from build123d import *

# Parameters (mm, degrees)
SKETCH1_R           = 50
SKETCH1_R_2         = 40
BOSS_EXTRUDE1_DEPTH = 10
SKETCH2_R           = 2
BOSS_EXTRUDE2_DEPTH = 33
CIRPATTERN1_COUNT   = 4


with BuildPart() as part:
    # Sketch1 → Boss-Extrude1 (new body)
    with BuildSketch(Plane(origin=(0, 0, 0), x_dir=(1, 0, 0), z_dir=(0, 1, 0))):
        with Locations(Location((0, 0, 0), (0, 0, 270))):
            Circle(SKETCH1_R)
        with Locations(Location((0, 0, 0), (0, 0, 270))):
            Circle(SKETCH1_R_2, mode=Mode.SUBTRACT)
    extrude(amount=BOSS_EXTRUDE1_DEPTH)

    # Sketch2 → Boss-Extrude2 (add)
    with BuildSketch(Plane(origin=(0, 10, 0), x_dir=(1, 0, 0), z_dir=(0, 1, 0))):
        with Locations(Location((0, 45, 0), (0, 0, 270))):
            Circle(SKETCH2_R)
    boss_extrude2 = extrude(amount=BOSS_EXTRUDE2_DEPTH)

    # CirPattern1: Boss-Extrude2 ×4 about axis
    cirpattern1_axis = Axis((0, 0, 0), (0, 1, 0))
    for i in range(1, CIRPATTERN1_COUNT):
        add(boss_extrude2.rotate(cirpattern1_axis, i * 360 / CIRPATTERN1_COUNT))


solid = part.part
Geometry: final body of the model. Coordinates: model frame, mm. A direction names the side the tool comes from. Round coordinates to 2 decimals unless told otherwise and drop trailing zeros. Loops run counter-clockwise (first coordinate to the right, second up) from the corner with the lowest first, then second, coordinate; pieces in that order, holes last. Notation, with made-up numbers: M -36,41.5 L 8,41.5 A34 ccw 8,77.5 Z; hole C -6.5,-40 d6. An arc over 180 degrees is marked long. Put each result on its own line as item: value. Start each with the question number.
(1) Draft query along X for faces 1 (the face through (0, 43, -45)), 2 (the face through (0, 26, 47)), 3 (the face through (-47, 26, 0)). Return one class per face: +X half, -X half, draft (parallel to the pull), parting line (faces both ways), or undercut.
(2) Section query B-B (z = 0). Return loops of the section in (x, y).
(3) Material intervals for line 1 along X through (y, z) = (5, 0); line 2 along Y through (x, z) = (-21, -36); line 3 along Z through (x, y) = (-25.5, 6), sorted ascending. Write a range as [from, to].
(4) Set-up query: faces 4 (the face through (0, 26, -47)), 5 (the face through (-45, 43, 0)). Return all of +Z, -Z, +X, -X, +Y, -Y with unobstructed straight access to the full face (end or side cutting, diameter ignored); none if empty.
(5) Contact query for flat-ended pins moving along their axis: pin 1 Ø5 at (y, z) = (12, -22.5) entering from -X; pin 2 Ø12 at (x, z) = (2.5, -30) entering from -Y; pin 3 Ø4 at (y, z) = (6, 19.5) entering from +X. Output: stop coordinate, or through.
(6) Section query D-D (z = 27.5). Return loops of the section in (x, y).
(7) Section query C-C (y = 14.5). Return loops of the section in (x, z).
(8) Section query A-A (x = 0). Return loops of the section in (y, z).
Findings below:
1. face 1: draft
1. face 2: parting line
1. face 3: undercut
2. outline: M -50,0 L -40,0 L -40,10 L -43,10 L -43,43 L -47,43 L -47,10 L -50,10 Z; M 40,0 L 50,0 L 50,10 L 47,10 L 47,43 L 43,43 L 43,10 L 40,10 Z
3. line 1: x = [-50, -40], [40, 50]
3. line 2: y = [0, 10]
3. line 3: z = [-43.01, -30.82], [30.82, 43.01]
4. face 4: +Y
4. face 5: +Z, -Z, +X, -X, +Y
5. pin 1: stops at x = -45.38
5. pin 2: passes through
5. pin 3: stops at x = 46.84
6. outline: M -41.76,0 L -29.05,0 L -29.05,10 L -41.76,10 Z; M 29.05,0 L 41.76,0 L 41.76,10 L 29.05,10 Z
7. outline: C -45,0 d4; C 0,-45 d4; C 0,45 d4; C 45,0 d4
8. outline: M 0,-50 L 10,-50 L 10,-47 L 43,-47 L 43,-43 L 10,-43 L 10,-40 L 0,-40 Z; M 0,40 L 10,40 L 10,43 L 43,43 L 43,47 L 10,47 L 10,50 L 0,50 Z
